Can you work these out from the model? Positions are in its coordinate system, mm. Face numbers are marked on the shaded views. A direction names the side the tool comes from. Coordinates: 2 decimals unless noted, no trailing zeros. Write each loop counter-clockwise with the first axis right and the second up, starting at its lowest first coordinate (ties: lowest second). Pieces come first, ordered by that corner, then holes.
```python
from build123d import *

# Parameters (mm, degrees)
F1_DEPTH = 15
F2_W     = 20
F2_H     = 55.2012861603
F3_DEPTH = 13
F4_R     = 2
F5_DEPTH = 10
F6_R     = 2.5
F8_DEPTH = 14.259891975
F9_DEPTH = 1.2510001


with BuildPart() as f1:
    # F0 (on Front) → F1 (new body, symmetric)
    with BuildSketch(Plane.XZ):
        with BuildLine():
            Line((20, 48.741108125), (20, 59.741108125))
            ThreePointArc((20, 59.741108125), (0, 63), (-20, 59.741108125))
            Line((-20, 59.741108125), (-20, 48.741108125))
            Line((-20, 48.741108125), (20, 48.741108125))
        make_face()
    extrude(amount=F1_DEPTH, both=True)

    # F2 (on Front) → F3 (cut, symmetric)
    with BuildSketch(Plane.XZ):
        with Locations((0, 27.6006430802)):
            Rectangle(F2_W, F2_H)
    extrude(amount=F3_DEPTH, both=True, mode=Mode.SUBTRACT)

    # F4 (on face) → F5 (cut)
    with BuildSketch(Plane(origin=(0, 0, 48.741108125), x_dir=(1, 0, 0), z_dir=(0, 0, -1))):
        with Locations((-15, 0)):
            Circle(F4_R)
        with Locations((15, 0)):
            Circle(F4_R)
    extrude(amount=-F5_DEPTH, mode=Mode.SUBTRACT)

    # F6
    f6_edges = [f1.edges().sort_by_distance(p)[0] for p in [
        (-20, -15, 54.241108),
        (-20, 15, 54.241108),
        (20, -15, 54.241108),
        (20, 15, 54.241108),
        (20, 0, 59.741108),
        (0, -15, 63),
        (0, 15, 63),
        (-20, 0, 59.741108),
    ]]
    fillet(f6_edges, radius=F6_R)

    # F7 (on face) → F8 (cut, through all)
    with BuildSketch(Plane(origin=(0, 0, 48.741108125), x_dir=(1, 0, 0), z_dir=(0, 0, -1))):
        with BuildLine():
            Line((17.5, 15), (-17.5, 15))
            ThreePointArc((-17.5, 15), (-19.267766953, 14.267766953), (-20, 12.5))
            Line((-20, 12.5), (-20, -12.5))
            ThreePointArc((-20, -12.5), (-19.267766953, -14.267766953), (-17.5, -15))
            Line((-17.5, -15), (17.5, -15))
            ThreePointArc((17.5, -15), (19.267766953, -14.267766953), (20, -12.5))
            Line((20, -12.5), (20, 12.5))
            ThreePointArc((20, 12.5), (19.267766953, 14.267766953), (17.5, 15))
        make_face()
        with BuildLine():
            Line((-19.25, -12.5), (-19.25, 12.5))
            ThreePointArc((-19.25, 12.5), (-18.7374368671, 13.7374368671), (-17.5, 14.25))
            Line((-17.5, 14.25), (17.5, 14.25))
            ThreePointArc((17.5, 14.25), (18.7374368671, 13.7374368671), (19.25, 12.5))
            Line((19.25, 12.5), (19.25, -12.5))
            ThreePointArc((19.25, -12.5), (18.7374368671, -13.7374368671), (17.5, -14.25))
            Line((17.5, -14.25), (-17.5, -14.25))
            ThreePointArc((-17.5, -14.25), (-18.7374368671, -13.7374368671), (-19.25, -12.5))
        make_face(mode=Mode.SUBTRACT)
    extrude(amount=-F8_DEPTH, mode=Mode.SUBTRACT)

    # F9 (cut, through all): a face of the model
    f9_faces = [f1.faces().sort_by_distance(p)[0] for p in [
        (0, -13, 51.9711971427),
    ]]
    extrude(f9_faces, amount=-F9_DEPTH, mode=Mode.SUBTRACT)


solid = f1.part
```
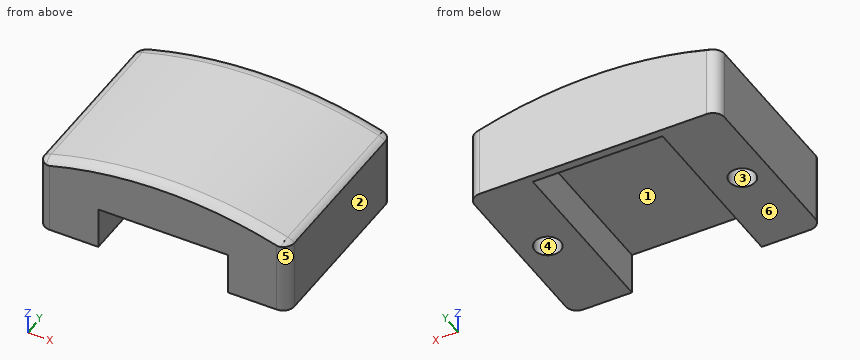
1. If I drill on L1, parallel to X at y = 0, z = 56; L2, parallel to X at y = 0, z = 52; L3, parallel to Y at x = -15, z = 54, over which ranges is the centre line in solid material (lowest first)?
2. If we section it at B-B, the plane y = 5.5: List the corners of the cut face in (x, z) for me.
3. If we section it at C-C, the plane x = 0: List the corners of the cut face in (y, z) for me.
4. If we section it at D-D, the plane y = 0.75: List the corners of the cut face in (x, z) for me, plus the area to 3 significant figures.
5. We'd pull the mould along X, two halves only. Please class the marked faces 4, 5 and 6: released by +X, released by -X, zero draft, split by the parting line, or undercut.
6. Which directions (+Z, -Z, +X, -X, +Y, -Y) give clear straight access to the entire face, cutting with the end or side of a thin tool? Please do the marked faces 1, 2 and 3.
7. I'm going to push flat-ended pins straight in: P1, Ø6, axis at x = -4, y = -7.5, coming from the -Z side; P2, Ø1.9, axis at x = -3, z = 52.5, coming from the -Y side; P3, Ø1, axis at x = 12, y = -7.5, coming from the +Z side; P4, Ø3, axis at x = -15.5, y = 1, coming from the -Z side. Where does each tip first touch, or does it pass through?
8. If we section it at A-A, the plane z = 53.5: List the corners of the cut face in (x, y) for me.
Answers:
1. L1: x = -19.25 to -17, -13 to 13, 17 to 19.25
1. L2: x = -19.25 to -17, -13 to -10, 10 to 13, 17 to 19.25
1. L3: y = -14.25 to -2, 2 to 14.25
2. outline: (-19.25, 48.74) - (-10, 48.74) - (-10, 55.2) - (10, 55.2) - (10, 48.74) - (19.25, 48.74) - (19.25, 59.7) arc R2.5 ccw to (18.22, 60.31) arc R63 ccw to (-18.22, 60.31) arc R2.5 ccw to (-19.25, 59.7) - close
3. outline: (-14.25, 55.2) - (13, 55.2) - (13, 48.74) - (14.25, 48.74) - (14.25, 62.29) arc R2.5 ccw to (12.5, 63) - (-12.5, 63) arc R2.5 ccw to (-14.25, 62.29) - close
4. outline: (-19.25, 48.74) - (-16.85, 48.74) - (-16.85, 58.74) - (-13.15, 58.74) - (-13.15, 48.74) - (-10, 48.74) - (-10, 55.2) - (10, 55.2) - (10, 48.74) - (13.15, 48.74) - (13.15, 58.74) - (16.85, 58.74) - (16.85, 48.74) - (19.25, 48.74) - (19.25, 59.7) arc R2.5 ccw to (18.22, 60.31) arc R63 ccw to (-18.22, 60.31) arc R2.5 ccw to (-19.25, 59.7) - close
4. area: 307 mm2
5. face 4: undercut
5. face 5: released by +X
5. face 6: zero draft
6. face 1: -Z, -Y
6. face 2: +Z, -Z, +X, +Y, -Y
6. face 3: -Z
7. P1: stops at z = 55.2
7. P2: stops at y = 13
7. P3: stops at z = 61.94
7. P4: stops at z = 48.74
8. outline: (-19.25, -12.5) arc R1.75 ccw to (-17.5, -14.25) - (-10, -14.25) - (-10, 13) - (10, 13) - (10, -14.25) - (17.5, -14.25) arc R1.75 ccw to (19.25, -12.5) - (19.25, 12.5) arc R1.75 ccw to (17.5, 14.25) - (-17.5, 14.25) arc R1.75 ccw to (-19.25, 12.5) - close; hole circle Ø4 at (-15, 0); hole circle Ø4 at (15, 0)
